Autodesk Inventor part; units mm, degrees
ref_plane "YZ Plane" through (0, 0, 0) normal (1, 0, 0) x (0, 1, 0)
ref_plane "XZ Plane" through (0, 0, 0) normal (0, 1, 0) x (-1, 0, 0)
ref_plane "XY Plane" through (0, 0, 0) normal (0, 0, 1) x (1, 0, 0)
sketch "Szkic2" plane through (0, 0, 0) normal (0, 1, 0) x (-1, 0, 0)
  line L0 (-11, 6) -> (11, 6)
  line L1 (11, 6) -> (11, -6)
  line L2 (11, -6) -> (-11, -6)
  line L3 (-11, -6) -> (-11, 6)
  line L4 (-11, 6) -> (11, -6) construction
  line L5 (11, 6) -> (-11, -6) construction
  line L6 (-11, 0) -> (-5, 0)
  circle A0 centre (-5, 0) radius 5
  line L7 (11, 0) -> (11, 2)
  line L8 (11, 2) -> (3, 2)
  line L9 (3, 2) -> (3, 6)
  line L10 (11, -6) -> (11, 6)
  line L11 (11, -2) -> (3, -2)
  line L12 (3, -2) -> (3, -6)
  point P0 (0, 0)
  point P1 (3, -6)
  point P2 (11, -2)
  dimension "d11" = 22
  dimension "d12" = 12
  dimension "d13" = 6
  dimension "d14" = 10
  dimension "d15" = 2
  dimension "d16" = 8
extrude "Wyciągnięcie proste3" add sketch "Szkic2" along normal blind 10 contours L0 L9 L8 L1 L11 L12 L2 L3
sketch "Szkic3" plane through (-11, 0, 2) normal (0, 0, 1) x (1, 0, 0)
  line L0 (0, 0) -> (0, 10)
  line L1 (8, 0) -> (0, 0)
  line L2 (0, 10) -> (0, 0)
  line L3 (8, 0) -> (8, 10)
  circle A0 centre (4, 5) radius 2
  point P0 (11, 0)
  dimension "d19" = 4
  dimension "d23" = 4
extrude "Wyciągnięcie proste4" cut sketch "Szkic3" against normal blind 32.75
fillet "Zaokrąglenie1" radius 5 6 edges at (-11, 0, 0) (-11, 10, 0) (-3, 0, 4) (-3, 10, 4) (-3, 0, -4) (-3, 10, -4)
properties part number "Knee"
Check sheet for the modelled part. Datum: model origin and axes. Units: mm. A direction names the side the tool comes from. Round coordinates to 2 decimals unless told otherwise and drop trailing zeros. Order: outer loops, then holes, each group sorted by start corner. A loop starts at its lowest first (then second) coordinate and runs counter-clockwise, first axis right, second up. Notation, with made-up numbers: M 80,-1 L 137,-1 A12 cw 137,3 Z; hole C 8.25,-22.5 d3. An arc over 180 degrees is marked long. One line per item, written item: value. Start each with the question number.
1. Section check C-C on x = 5. Enter the section's corners in (y, z).
2. Access from +Z, -Z, +X, -X, +Y, -Y to the whole of each face (thin tool, end or side, straight path). Record for faces 5 (the cylindrical face through (-3, 5, -4)), 6 (the flat face through (11, 5, 0)).
3. Section check A-A on y = 5. Enter the section's corners in (x, z), and give its area (3 significant figures).
4. Scan lines: line 1 along X through (y, z) = (3.25, 1.75); line 2 along Z through (x, y) = (5, 5.25); line 3 along X through (y, z) = (5.75, 0). Record each from-to range of solid material in increasing order.
5. Section check D-D on x = -2. Enter the section's corners in (y, z), and give its area (3 significant figures).
6. Gauge pin test, flat ends, axial feed: P1, Ø2, axis at y = 1, z = -3.5, coming from the -X side; P2, Ø5, axis at x = -7, y = 5, coming from the -Z side. Record the tip position at first contact, or that the pin passes through.
7. Release check for a two-part mould opening along X. For faces 1 (the flat face through (-5, 6, 2)), 2 (the cylindrical face through (0.23, 4.93, -1.5)), 3 (the cylindrical face through (-9, 5, 0)), 4 (the cylindrical face through (-3, 5, 4)) record: released by +X, released by -X, zero draft, split by the parting line, or undercut.
Results found:
1. outline: M 0,-6 L 10,-6 L 10,-5 L 0,-5 Z; M 0,5 L 10,5 L 10,6 L 0,6 Z
2. face 5: -Z, -X
2. face 6: +Z, -Z, +X, +Y, -Y
3. outline: M -11,-2 L -9,-2 L -9,2 L -11,2 Z; M -5,-2 L -3,-2 L -3,-6 L 11,-6 L 11,6 L -3,6 L -3,2 L -5,2 Z; hole C 5,0 d10
3. area: 105 mm^2
4. line 1: -10.68 to -7.97, -6.03 to 0.32, 9.68 to 11
4. line 2: -6 to -5, 5 to 6
4. line 3: -10.94 to -8.85, -5.15 to 0, 10 to 11
5. outline: M 0,-2 L 2,-2 L 2,-6 L 8,-6 L 8,-2 L 10,-2 L 10,2 L 8,2 L 8,6 L 2,6 L 2,2 L 0,2 Z
5. area: 88.0 mm^2
6. P1: x = -2
6. P2: z = -2
7. face 1: zero draft
7. face 2: undercut
7. face 3: undercut
7. face 4: released by -X
